Design review of the part built by this model. Coordinates are the model's own, in mm. Face numbers are marked on the shaded views. A direction names the side the tool comes from. Give positions to 0.01 mm unless a question says otherwise; leave off trailing zeros. Order: outer loops, then holes, each group sorted by start corner. A loop starts at its lowest first (then second) coordinate and runs counter-clockwise, first axis right, second up. Notation, with made-up numbers: (-17.5, 50) -> (11.5, 50) arc R10 ccw to (11.5, 58) -> close; hole circle Ø8 at (83.5, -23.75). An arc over 180 degrees is marked (long way). Use a Markdown table: item, result. Add a question column.
```python
from build123d import *

# Parameters (mm, degrees)
F0_W      = 30
F0_H      = 23
F1_DEPTH  = 25
F2_W      = 25
F2_H      = 15
F3_DEPTH  = 15
F4_R      = 5
F5_DEPTH  = 25
F6_R      = 7.5
F7_DEPTH  = 5
F8_W      = 40
F8_H      = 30
F9_DEPTH  = 30
F10_R     = 5.5
F11_DEPTH = 5
F12_R     = 2.5
F13_DEPTH = 5
F14_R     = 2.5
F15_DEPTH = 5


with BuildPart() as f1:
    # F0 (on Top) → F1 (new body)
    with BuildSketch(Plane.XY):
        Rectangle(F0_W, F0_H)
    extrude(amount=F1_DEPTH)

    # F2 (on face) → F3 (join)
    with BuildSketch(Plane(origin=(0, 0, 0), x_dir=(1, 0, 0), z_dir=(0, 0, -1))):
        Rectangle(F2_W, F2_H)
    extrude(amount=F3_DEPTH)

    # F4 (on face) → F5 (join)
    with BuildSketch(Plane(origin=(0, 0, -15), x_dir=(1, 0, 0), z_dir=(0, 0, -1))):
        with Locations((7, 0)):
            Circle(F4_R)
        with Locations((-7, 0)):
            Circle(F4_R)
    extrude(amount=F5_DEPTH)

    # F6 (on face) → F7 (join)
    with BuildSketch(Plane.XY.offset(25)):
        Circle(F6_R)
    extrude(amount=F7_DEPTH)

    # F8 (on face) → F9 (join)
    with BuildSketch(Plane.XY.offset(30)):
        Rectangle(F8_W, F8_H)
    extrude(amount=F9_DEPTH)

    # F10 (on face) → F11 (cut)
    with BuildSketch(Plane.XZ.offset(15)):
        with Locations((-11, 45)):
            Circle(F10_R)
        with Locations((11, 45)):
            Circle(F10_R)
    extrude(amount=-F11_DEPTH, mode=Mode.SUBTRACT)

    # F12 (on face) → F13 (join)
    with BuildSketch(Plane.XZ.offset(10)):
        with Locations((-11, 45)):
            Circle(F12_R)
    extrude(amount=F13_DEPTH)

    # F14 (on face) → F15 (join)
    with BuildSketch(Plane.XZ.offset(10)):
        with Locations((11, 45)):
            Circle(F14_R)
    extrude(amount=F15_DEPTH)


solid = f1.part
```
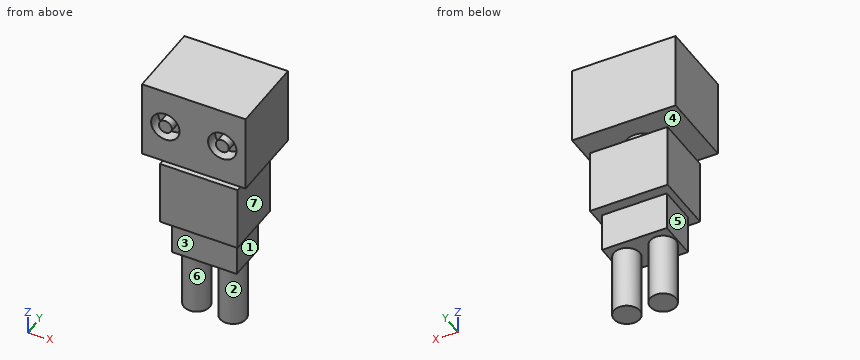
1) Add section C-C (y = 0). Give the boundary of the cut face in (x, z).
2) Add section B-B (z = 45). Give the boundary of the cut face in (x, y).
3) Insertion check: pin 1 (5 mm diameter, centred on y = 5, z = -24, fed in from +X); pin 2 (8 mm diameter, centred on y = 11.5, z = 6, fed in from -X); pin 3 (10 mm diameter, centred on y = 5, z = -29, fed in from +X); pin 4 (4 mm diameter, centred on y = 10, z = -10.5, fed in from +X). Each pin has a flat end and moves straight along its axis. Give the tip position at first contact, or say it passes through.
4) For L1, parallel to Z at x = 11, y = -11.7; L2, parallel to Z at x = 11, y = -11.45; L3, parallel to X at y = -10.5, z = 43, list the stretches that pass through material, from the lowest coordinate up. Write a range as [from, to].
5) Add section D-D (x = 0). Give the boundary of the cut face in (y, z).
6) The part is to be moulded in two halves that separate along X. For the marked faces 4, 5, 6 and 7, say which applies: +X half, -X half, draft (parallel to the pull), parting line (faces both ways), or undercut.
7) Machinability: for the marked faces 1, 2 and 3, which of the approach directions +Z, -Z, +X, -X, +Y, -Y give a long, thin tool a straight path to every point of the face, cutting with its end or side? Answer none if there is none.
8) Add section A-A (x = 11). Give the boundary of the cut face in (y, z), then the cut area to 3 significant figures.
Worked answers:
| question | item | result |
|---|---|---|
| 1 | outline | (-20, 30) -> (-7.5, 30) -> (-7.5, 25) -> (-15, 25) -> (-15, 0) -> (-12.5, 0) -> (-12.5, -15) -> (-12, -15) -> (-12, -40) -> (-2, -40) -> (-2, -15) -> (2, -15) -> (2, -40) -> (12, -40) -> (12, -15) -> (12.5, -15) -> (12.5, 0) -> (15, 0) -> (15, 25) -> (7.5, 25) -> (7.5, 30) -> (20, 30) -> (20, 60) -> (-20, 60) -> close |
| 2 | outline | (-20, -15) -> (-16.5, -15) -> (-16.5, -10) -> (-13.5, -10) -> (-13.5, -15) -> (-8.5, -15) -> (-8.5, -10) -> (-5.5, -10) -> (-5.5, -15) -> (5.5, -15) -> (5.5, -10) -> (8.5, -10) -> (8.5, -15) -> (13.5, -15) -> (13.5, -10) -> (16.5, -10) -> (16.5, -15) -> (20, -15) -> (20, 15) -> (-20, 15) -> close |
| 3 | pin 1 | x = 11.33 |
| 3 | pin 2 | x = -15 |
| 3 | pin 3 | x = 12 |
| 3 | pin 4 | through |
| 4 | L1 | [30, 39.5], [42.5, 47.5], [50.5, 60] |
| 4 | L2 | [0, 25], [30, 39.5], [42.5, 47.5], [50.5, 60] |
| 4 | L3 | [-20, -16.12], [-12.5, -9.5], [-5.88, 5.88], [9.5, 12.5], [16.12, 20] |
| 5 | outline | (-15, 30) -> (-7.5, 30) -> (-7.5, 25) -> (-11.5, 25) -> (-11.5, 0) -> (-7.5, 0) -> (-7.5, -15) -> (7.5, -15) -> (7.5, 0) -> (11.5, 0) -> (11.5, 25) -> (7.5, 25) -> (7.5, 30) -> (15, 30) -> (15, 60) -> (-15, 60) -> close |
| 6 | face 4 | draft |
| 6 | face 5 | -X half |
| 6 | face 6 | undercut |
| 6 | face 7 | +X half |
| 7 | face 1 | -Z, +X, +Y, -Y |
| 7 | face 2 | -Z |
| 7 | face 3 | -Z, +X, -X, -Y |
| 8 | outline | (-15, 30) -> (15, 30) -> (15, 60) -> (-15, 60) -> (-15, 50.5) -> (-10, 50.5) -> (-10, 47.5) -> (-15, 47.5) -> (-15, 42.5) -> (-10, 42.5) -> (-10, 39.5) -> (-15, 39.5) -> close; (-11.5, 0) -> (-7.5, 0) -> (-7.5, -15) -> (-3, -15) -> (-3, -40) -> (3, -40) -> (3, -15) -> (7.5, -15) -> (7.5, 0) -> (11.5, 0) -> (11.5, 25) -> (-11.5, 25) -> close |
| 8 | area | 1,820 mm^2 |
